Autodesk Fusion 360 part; units mm, degrees
sketch "Sketch1" plane through (0, 0, 0) normal (0, 1, 0) x (1, 0, 0) in component "Case"
  line L0 (0, 0) -> (84, 0)
  line L1 (84, 0) -> (84, -104)
  line L2 (84, -104) -> (0, -104)
  line L3 (0, -104) -> (0, 0)
  dimension "d1" = 84
  dimension "d2" = 104
extrude "Extrude1" add sketch "Sketch1" along normal blind 32 in component "Case"
shell "Shell1" thickness 2 removed faces 1 at (56, 10.6667, 104) in component "Case"
fillet "Fillet1" radius 1 4 edges at (0, 16, 104) (42, 32, 104) (84, 16, 104) (42, 0, 104) in component "Case"
sketch "Sketch2" plane through (84, 0, 0) normal (1, 0, 0) x (0, 1, 0) in component "Case"
  line L0 (32, 103) -> (0, 103)
  line L1 (0, 103) -> (0, 0)
  line L2 (0, 0) -> (32, 0)
  line L3 (32, 0) -> (32, 103)
  line L4 (0, 0) -> (32, 0)
  line L5 (32, 0) -> (32, 60)
  line L6 (32, 60) -> (0, 60)
  line L7 (0, 60) -> (0, 0)
  dimension "d8" = 60
extrude "Extrude2" cut sketch "Sketch2" against normal blind 5 contours L1 L2 L3 L4 L5 L6 L7 in component "Case"
sketch "Sketch3" plane through (0, 0, 0) normal (-1, 0, 0) x (0, -1, 0) in component "Case"
  line L0 (0, 103) -> (-32, 103)
  line L1 (-32, 103) -> (-32, 0)
  line L2 (-32, 0) -> (0, 0)
  line L3 (0, 0) -> (0, 103)
  line L4 (0, 0) -> (-32, 0)
  line L5 (-32, 0) -> (-32, 60)
  line L6 (-32, 60) -> (0, 60)
  line L7 (0, 60) -> (0, 0)
  dimension "d11" = 60
extrude "Extrude3" cut sketch "Sketch3" against normal blind 5 contours L1 L2 L3 L4 L5 L6 L7 in component "Case"
sketch "Sketch4" plane through (0, 32, 0) normal (0, 1, 0) x (-1, 0, 0) in component "Case"
  line L0 (-5, 60) -> (0, 60)
  line L1 (0, 60) -> (0, 103)
  line L2 (0, 103) -> (-84, 103)
  line L3 (-84, 103) -> (-84, 60)
  line L4 (-84, 60) -> (-79, 60)
  line L5 (-79, 60) -> (-79, 0)
  line L6 (-79, 0) -> (-5, 0)
  line L7 (-5, 0) -> (-5, 60)
  line L8 (-70, 85) -> (-15, 85)
  line L9 (-15, 85) -> (-15, 10)
  line L10 (-15, 10) -> (-70, 10)
  line L11 (-70, 10) -> (-70, 85)
  line L12 (-70, 85) -> (-15, 85)
  line L13 (-15, 85) -> (-15, 10)
  line L14 (-15, 10) -> (-70, 10)
  line L15 (-70, 10) -> (-70, 85)
extrude "Extrude4" cut sketch "Sketch4" against normal blind 5 contours L8 L9 L10 L11 L12 L13 L14 L15 in component "Case"
sketch "Sketch5" plane through (0, 0, 0) normal (0, -1, 0) x (1, 0, 0) in component "Case"
  line L0 (0, 60) -> (5, 60)
  line L1 (5, 60) -> (5, 0)
  line L2 (5, 0) -> (79, 0)
  line L3 (79, 0) -> (79, 60)
  line L4 (79, 60) -> (84, 60)
  line L5 (84, 60) -> (84, 103)
  line L6 (84, 103) -> (0, 103)
  line L7 (0, 103) -> (0, 60)
  circle A0 centre (25, 75) radius 2.5
  circle A1 centre (60, 75) radius 2.5
  dimension "d16" = 5
  dimension "d17" = 5
extrude "Extrude5" cut sketch "Sketch5" against normal blind 5 contours A0 | A1 in component "Case"
sketch "Sketch6" plane through (0, 0, 0) normal (0, -1, 0) x (1, 0, 0) in component "Case"
  circle A0 centre (25, 75) radius 2.5
  circle A1 centre (60, 75) radius 2.5
  line L0 (0, 60) -> (5, 60)
  line L1 (5, 60) -> (5, 0)
  line L2 (5, 0) -> (79, 0)
  line L3 (79, 0) -> (79, 60)
  line L4 (79, 60) -> (84, 60)
  line L5 (84, 60) -> (84, 103)
  line L6 (84, 103) -> (0, 103)
  line L7 (0, 103) -> (0, 60)
  circle A2 centre (25, 25) radius 2.5
  circle A3 centre (60, 25) radius 2.5
extrude "Extrude6" cut sketch "Sketch6" against normal blind 5 contours A2 | A3 in component "Case"
component "Case" placed x (1, 0, 0) y (0, 1, 0) z (0, 0, 1) at (0, 0, 0)
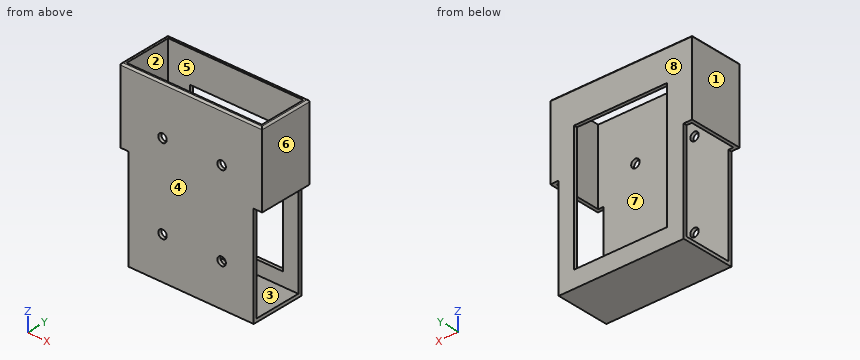
Source: CAD feature listing. Evaluate the final solid. Frame: model axes, mm. Face numbers are marked on the shaded views. A direction names the side the tool comes from. Coordinates: 2 decimals unless noted, no trailing zeros. Loops run counter-clockwise (first coordinate to the right, second up) from the corner with the lowest first, then second, coordinate; pieces in that order, holes last. Notation, with made-up numbers: (-5.75, -14) - (52.25, -14) arc R19 cw to (52.25, 22) - close; hole circle Ø3 at (71.25, 77.25). An arc over 180 degrees is marked (long way). One line per item, written item: value. Start each with the question number.
1. Ray query, L1, parallel to Z at x = 60, y = 1; L2, parallel to Y at x = 68, z = 99.5; L3, parallel to X at y = 13, z = 84. Return the intervals inside material, ascending.
2. Set-up query: the marked faces 1, 2, 3, 4 and 5. Return all of +Z, -Z, +X, -X, +Y, -Y with unobstructed straight access to the full face (end or side cutting, diameter ignored); none if empty.
3. Section B-B (z = 25). Return the cut outline in (x, y), and give its area (3 significant figures).
4. Section A-A (z = 43). Return the cut outline in (x, y).
5. Section D-D (y = 18.5). Return the cut outline in (x, z), and give its area (3 significant figures).
6. Mould query, pull axis Y, two halves, no side actions, for the marked faces 6, 7 and 8. Classes: pulls with the +Y half, pulls with the -Y half, needs draft (parallel to the pull), parting line crosses it, or undercut.
7. Section C-C (x = 54). Return the cut outline in (y, z), and give its area (3 significant figures).
8. Contact query for flat-ended pins moving along their axis: P1, Ø0.6, axis at y = 31.5, z = 45.5, coming from the +X side; P2, Ø1.5, axis at x = 11.5, y = 10, coming from the +Z side; P3, Ø2, axis at y = 31, z = 57, coming from the -X side. Output: stop coordinate, or through.
Verdict:
1. L1: z = 0 to 22.5, 27.5 to 72.5, 77.5 to 104
1. L2: y = 0 to 2, 30 to 32
1. L3: x = 0 to 2, 82 to 84
2. face 1: +Z, -Z, -X, +Y, -Y
2. face 2: +Z, -Z
2. face 3: +Z, +X, -X
2. face 4: +Z, -Z, +X, -X, -Y
2. face 5: +Z
3. outline: (5, 0) - (22.5, 0) - (22.5, 2) - (5, 2) - close; (5, 30) - (15, 30) - (15, 32) - (5, 32) - close; (27.5, 0) - (57.5, 0) - (57.5, 2) - (27.5, 2) - close; (62.5, 0) - (79, 0) - (79, 2) - (62.5, 2) - close; (70, 30) - (79, 30) - (79, 32) - (70, 32) - close
3. area: 166 mm2
4. outline: (5, 0) - (79, 0) - (79, 2) - (5, 2) - close; (5, 30) - (15, 30) - (15, 32) - (5, 32) - close; (70, 30) - (79, 30) - (79, 32) - (70, 32) - close
5. outline: (0, 60) - (2, 60) - (2, 104) - (1, 104) arc R1 ccw to (0, 103) - close; (5, 0) - (79, 0) - (79, 2) - (5, 2) - close; (82, 60) - (84, 60) - (84, 103) arc R1 ccw to (83, 104) - (82, 104) - close
5. area: 324 mm2
6. face 6: needs draft
6. face 7: undercut
6. face 8: pulls with the +Y half
7. outline: (0, 0) - (32, 0) - (32, 10) - (30, 10) - (30, 2) - (2, 2) - (2, 104) - (1, 104) arc R1 ccw to (0, 103) - close; (30, 85) - (32, 85) - (32, 103) arc R1 ccw to (31, 104) - (30, 104) - close
7. area: 322 mm2
8. P1: stops at x = 79
8. P2: stops at z = 2
8. P3: stops at x = 5
